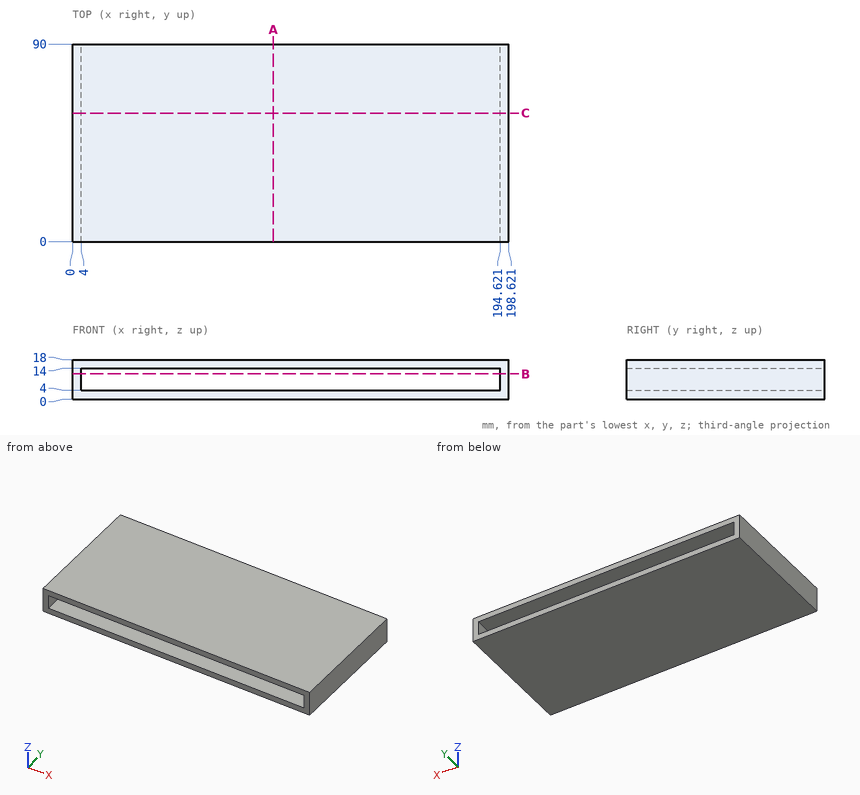
Check sheet for the drawn part. Datum: minimum x, y, z corner. Units: mm. Round coordinates to 2 decimals unless told otherwise and drop trailing zeros. Order: outer loops, then holes, each group sorted by start corner. A loop starts at its lowest first (then second) coordinate and runs counter-clockwise, first axis right, second up.
(1) Cross-section at C-C, the plane y = 58.5. Enter the section's corners in (x, z), and give its area (3 significant figures).
(2) Cross-section at B-B, the plane z = 11.5. Enter the section's corners in (x, y), and give its area (3 significant figures).
(3) Cross-section at A-A, the plane x = 91.5. Enter the section's corners in (y, z), and give its area (3 significant figures).
(4) Scan lines: probe 1 along Z at (x, y) = (142, 18.5); probe 2 along X at (y, z) = (57, 8.25). Record each from-to range of solid material in increasing order.
Check sheet entries:
1. outline: (0, 0) - (198.62, 0) - (198.62, 18) - (0, 18) - close; hole (4, 4) - (194.62, 4) - (194.62, 14) - (4, 14) - close
1. area: 1,670 mm2
2. outline: (0, 0) - (4, 0) - (4, 90) - (0, 90) - close; (194.62, 0) - (198.62, 0) - (198.62, 90) - (194.62, 90) - close
2. area: 720 mm2
3. outline: (0, 0) - (90, 0) - (90, 4) - (0, 4) - close; (0, 14) - (90, 14) - (90, 18) - (0, 18) - close
3. area: 720 mm2
4. probe 1: z = 0 to 4, 14 to 18
4. probe 2: x = 0 to 4, 194.62 to 198.62
